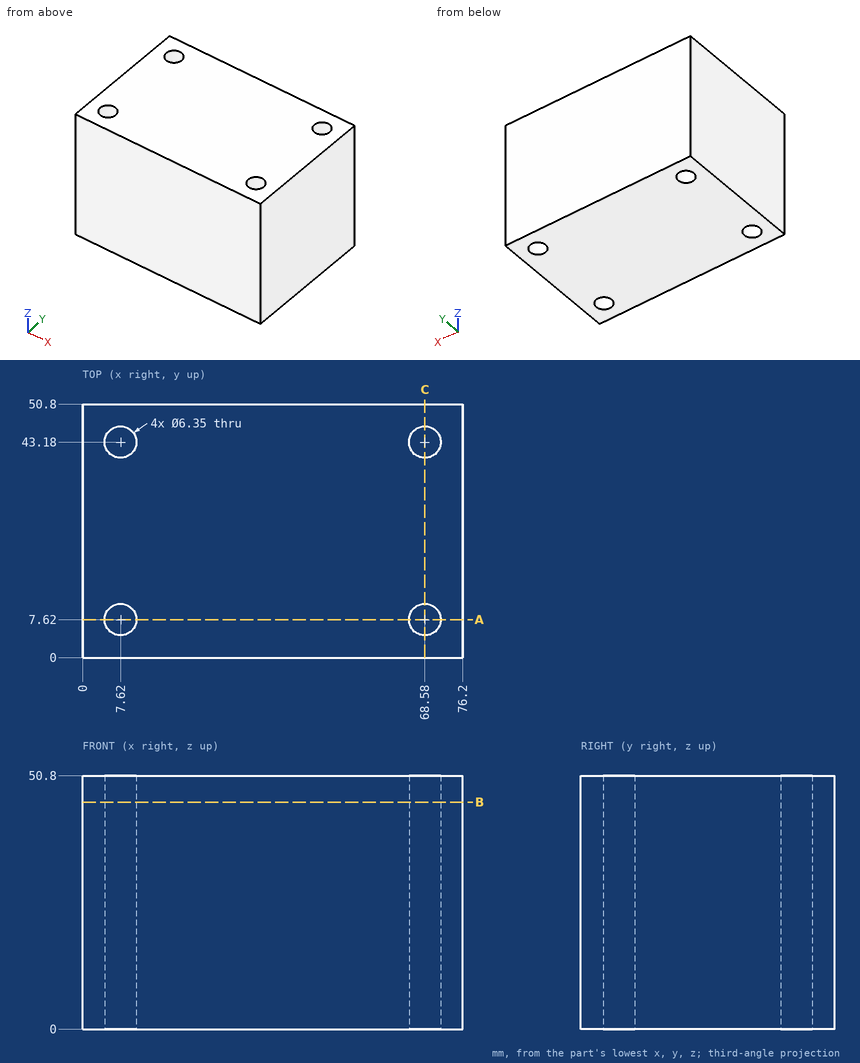
Check sheet for the drawn part. Datum: minimum x, y, z corner. Units: mm. Coordinates: 2 decimals unless noted, no trailing zeros. Loops run counter-clockwise (first coordinate to the right, second up) from the corner with the lowest first, then second, coordinate; pieces in that order, holes last. Notation, with made-up numbers: (81.5, 35) -> (92.5, 35) arc R19 cw to (92.5, 47) -> close; hole circle Ø8 at (2, -12). An arc over 180 degrees is marked (long way). Answer as a JSON object with one key per item and string values. Group by question number.
Item 1: Scan lines: probe 1 along Y at (x, z) = (7.62, 40) (3 decimals); probe 2 along X at (y, z) = (6, 33); probe 3 along X at (y, z) = (7, 34). Record each from-to range of solid material in increasing order.
Item 2: Sectioned sample at C-C on x = 68.58. Record the boundary of the cut face in (y, z) (3 decimals).
Item 3: Sectioned sample at B-B on z = 45.5. Record the boundary of the cut face in (x, y) (3 decimals).
Item 4: Sectioned sample at A-A on y = 7.62. Record the boundary of the cut face in (x, z) (3 decimals).
Evaluation:
{
 "1": {"probe 1": "y = 0 to 4.445, 10.795 to 40.005, 46.355 to 50.8", "probe 2": "x = 0 to 4.89, 10.35 to 65.85, 71.31 to 76.2", "probe 3": "x = 0 to 4.51, 10.73 to 65.47, 71.69 to 76.2"},
 "2": {"outline": "(0, 0) -> (4.445, 0) -> (4.445, 50.8) -> (0, 50.8) -> close; (10.795, 0) -> (40.005, 0) -> (40.005, 50.8) -> (10.795, 50.8) -> close; (46.355, 0) -> (50.8, 0) -> (50.8, 50.8) -> (46.355, 50.8) -> close"},
 "3": {"outline": "(0, 0) -> (76.2, 0) -> (76.2, 50.8) -> (0, 50.8) -> close; hole circle Ø6.35 at (7.62, 7.62); hole circle Ø6.35 at (7.62, 43.18); hole circle Ø6.35 at (68.58, 7.62); hole circle Ø6.35 at (68.58, 43.18)"},
 "4": {"outline": "(0, 0) -> (4.445, 0) -> (4.445, 50.8) -> (0, 50.8) -> close; (10.795, 0) -> (65.405, 0) -> (65.405, 50.8) -> (10.795, 50.8) -> close; (71.755, 0) -> (76.2, 0) -> (76.2, 50.8) -> (71.755, 50.8) -> close"}
}
